Answer from the drawing. Dimensions are ordinates in mm from the lowest x, y and z of the part. A direction names the side the tool comes from. Round coordinates to 2 decimals unless told otherwise and drop trailing zeros. Order: outer loops, then holes, each group sorted by start corner. A loop starts at its lowest first (then second) coordinate and runs counter-clockwise, first axis right, second up. Notation, with made-up numbers: (-30.5, 0.5) -> (-9.5, 0.5) arc R33 ccw to (-9.5, 37.5) -> close; hole circle Ø6 at (-1, 59.5). An arc over 180 degrees is marked (long way). Use a Markdown table: item, result. Add a question column.
Item 1: A tool of negligible diameter and unlimited length cuts with its end or side. For the marked faces 1 and 2, from which of +Z, -Z, +X, -X, +Y, -Y can it reach the whole face along a straight path? Write none if from no direction.
Item 2: For a pull along X with two mould halves and no side action, classify the marked faces 3, 4, 5 and 6 as +X half, -X half, draft (parallel to the pull), parting line (faces both ways), or undercut.
Item 3: A cutting plane is placed at A-A, the plane x = 31. Determine the outline of the cut face in (y, z), plus the area to 3 significant figures.
Item 4: A cutting plane is placed at C-C, the plane z = 11. Determine the outline of the cut face in (x, y), plus the area to 3 significant figures.
Item 5: A cutting plane is placed at B-B, the plane y = 13. Determine the outline of the cut face in (x, z).
Item 6: Flat-ended cylindrical pins translate along their axes: P1, Ø2.5, axis at y = 2.5, z = 36.5, coming from the +X side; P2, Ø6, axis at x = 119.5, z = 51, coming from the -Y side; P3, Ø10, axis at x = 103, y = 67.5, coming from the +Z side. Find the tip coordinate at first contact, or state that the pin passes through.
Item 7: Find the intervals of material crossed by L1, parallel to X at y = 34, z = 50.5; L2, parallel to Z at x = 68.5, y = 65.5; L3, parallel to Y at x = 38, z = 9.5, in increasing order. Write a range as [from, to].
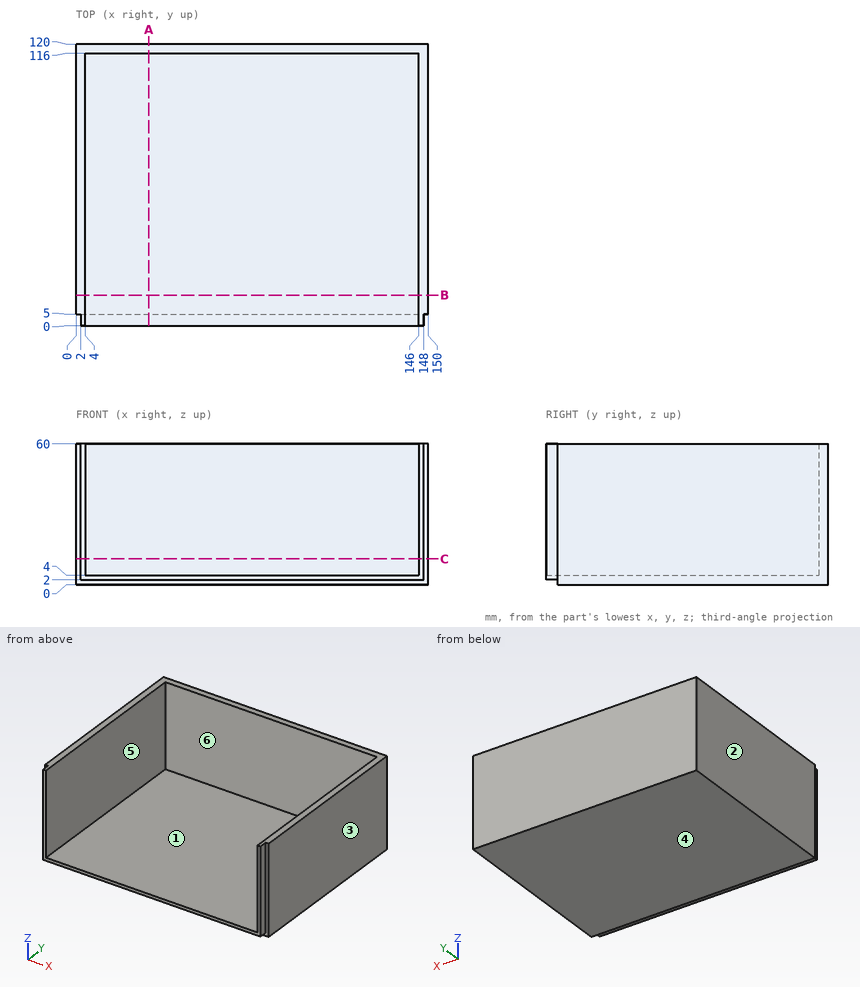
Reported:
| question | item | result |
|---|---|---|
| 1 | face 1 | +Z, -Y |
| 1 | face 2 | +Z, -Z, -X, +Y, -Y |
| 2 | face 3 | +X half |
| 2 | face 4 | draft |
| 2 | face 5 | undercut |
| 2 | face 6 | undercut |
| 3 | outline | (0, 2) -> (5, 2) -> (5, 0) -> (120, 0) -> (120, 60) -> (116, 60) -> (116, 4) -> (0, 4) -> close |
| 3 | area | 694 mm² |
| 4 | outline | (0, 5) -> (2, 5) -> (2, 0) -> (4, 0) -> (4, 116) -> (146, 116) -> (146, 0) -> (148, 0) -> (148, 5) -> (150, 5) -> (150, 120) -> (0, 120) -> close |
| 4 | area | 1,510 mm² |
| 5 | outline | (0, 0) -> (150, 0) -> (150, 60) -> (146, 60) -> (146, 4) -> (4, 4) -> (4, 60) -> (0, 60) -> close |
| 6 | P1 | x = 148 |
| 6 | P2 | y = 116 |
| 6 | P3 | z = 4 |
| 7 | L1 | [0, 4], [146, 150] |
| 7 | L2 | [0, 4] |
| 7 | L3 | [116, 120] |
